Input: part model. Units: mm. Frame: model coordinates. Face numbers are marked on the shaded views. A direction names the side the tool comes from. Round coordinates to 2 decimals unless told otherwise and drop trailing zeros. Loops run counter-clockwise (first coordinate to the right, second up) from the corner with the lowest first, then second, coordinate; pieces in that order, holes last.
(1) Cut plane A-A, the plane y = 22. Output: boundary loops of the cut face in (x, z), and give its area (3 significant figures).
(2) Line query: line 1 (X direction, y = 32.75, z = 5); line 2 (Z direction, x = 0, y = 39); line 3 (Y direction, x = -48, z = 10). Output: solid intervals per line, ascending.
(3) Draft query along Z for the marked faces 1, 2, 3 and 4. Return one class per face: released by +Z, released by -Z, zero draft, split by the parting line, or undercut.
(4) First-contact query: pin 1 Ø12.5 at (x, y) = (-34.5, 28) entering from -Z; pin 2 Ø3 at (x, z) = (-34.25, -5) entering from -Y; pin 3 Ø6.5 at (x, y) = (13.5, 17.5) entering from -Z. Flat tips, straight axial feed; report the tip coordinate or a pass-through.
(5) Cut plane C-C, the plane y = 7. Output: boundary loops of the cut face in (x, z), and give its area (3 significant figures).
(6) Access query for the marked faces 5 and 6. Directions: +Z, -Z, +X, -X, +Y, -Y. A direction counts if a zero-diameter tool reaches every point of the face in a straight line with its end or side. Return the directions, or none.
(7) Cut plane B-B, the plane x = 0. Output: boundary loops of the cut face in (y, z) (3 decimals).
(8) Cut plane D-D, the plane y = 51. Output: boundary loops of the cut face in (x, z).
from build123d import *

# Parameters (mm, degrees)
SKETCH1_R                                           = 60.625
SKETCH1_R_2                                         = 45
BOSS_EXTRUDE1_DEPTH                                 = 4
SKETCH2_R                                           = 49
SKETCH2_R_2                                         = 45
BOSS_EXTRUDE2_DEPTH                                 = 52
SKETCH4_W                                           = 13.25
SKETCH4_H                                           = 8
SKETCH4_W_2                                         = 8
SKETCH4_H_2                                         = 38
BOSS_EXTRUDE4_DEPTH                                 = 13
BOSS_EXTRUDE5_DEPTH                                 = 4
SKETCH7_R                                           = 1.3
CUT_EXTRUDE4_DEPTH                                  = 7.2
SKETCH9_W                                           = 10
SKETCH9_H                                           = 24
CUT_EXTRUDE7_DEPTH                                  = 8
CUT_EXTRUDE8_REACH                                  = 111.625
SKETCH11_R                                          = 5
CUT_EXTRUDE9_DEPTH                                  = 5.0000001
CSK_FOR_M3_COUNTERSUNK_FLAT_HEAD_SCREW1_D           = 3.4
CSK_FOR_M3_COUNTERSUNK_FLAT_HEAD_SCREW1_DEPTH       = 4
CSK_FOR_M3_COUNTERSUNK_FLAT_HEAD_SCREW1_CSINK_D     = 6.3
CSK_FOR_M3_COUNTERSUNK_FLAT_HEAD_SCREW1_CSINK_ANGLE = 90


with BuildPart() as part:
    # Sketch1 → Boss-Extrude1 (new body)
    with BuildSketch(Plane(origin=(0, 0, 0), x_dir=(1, 0, 0), z_dir=(0, 1, 0))):
        Circle(SKETCH1_R)
        Circle(SKETCH1_R_2, mode=Mode.SUBTRACT)
    extrude(amount=BOSS_EXTRUDE1_DEPTH)

    # Sketch2 → Boss-Extrude2 (add)
    with BuildSketch(Plane(origin=(0, 4, 0), x_dir=(1, 0, 0), z_dir=(0, 1, 0))):
        Circle(SKETCH2_R)
        Circle(SKETCH2_R_2, mode=Mode.SUBTRACT)
    extrude(amount=BOSS_EXTRUDE2_DEPTH)

    # Sketch4 → Boss-Extrude4 (add, symmetric)
    with BuildSketch(Plane.XY):
        with Locations((-38.375, 34)):
            Rectangle(SKETCH4_W, SKETCH4_H)
        Polygon((-31.75, 30), (-45, 30), (-45, 16.75), align=None)
        with Locations((15.25, 19)):
            Rectangle(SKETCH4_W_2, SKETCH4_H_2)
    extrude(amount=BOSS_EXTRUDE4_DEPTH, both=True)

    # Sketch5 → Boss-Extrude5 (add)
    with BuildSketch(Plane.XZ):
        with BuildLine():
            Line((11.25, 13), (29.067400866, 34.352382842))
            ThreePointArc((29.067400866, 34.352382842), (45, 0), (29.067400866, -34.352382842))
            Line((29.067400866, -34.352382842), (11.25, -13))
            Line((11.25, -13), (11.25, 13))
        make_face()
    extrude(amount=-BOSS_EXTRUDE5_DEPTH)

    # Sketch7 → Cut-Extrude4 (cut)
    with BuildSketch(Plane(origin=(0, 38, 0), x_dir=(1, 0, 0), z_dir=(0, 1, 0))):
        with Locations((-34.25, 5)):
            Circle(SKETCH7_R)
        with Locations((-34.25, -5)):
            Circle(SKETCH7_R)
        with Locations((13.75, 5)):
            Circle(SKETCH7_R)
        with Locations((13.75, -5)):
            Circle(SKETCH7_R)
    extrude(amount=-CUT_EXTRUDE4_DEPTH, mode=Mode.SUBTRACT)

    # Sketch9 → Cut-Extrude7 (cut)
    with BuildSketch(Plane.ZY.offset(-11.25)):
        with Locations((0, 17)):
            Rectangle(SKETCH9_W, SKETCH9_H)
    extrude(amount=-CUT_EXTRUDE7_DEPTH, mode=Mode.SUBTRACT)

    # Sketch11 → Cut-Extrude8 (cut, up to next)
    with BuildSketch(Plane(origin=(49, 0, 0), x_dir=(0, 0, -1), z_dir=(1, 0, 0)), mode=Mode.PRIVATE) as cut_extrude8_sk1:
        with Locations((0, 14)):
            Circle(SKETCH11_R)
    cut_extrude8_tool1 = extrude(cut_extrude8_sk1.sketch, amount=-CUT_EXTRUDE8_REACH, mode=Mode.PRIVATE) & part.part
    add(cut_extrude8_tool1.solids().sort_by_distance((49, 14, 0))[0], mode=Mode.SUBTRACT)

    # Sketch12 → Cut-Extrude9 (cut, through all)
    with BuildSketch(Plane(origin=(0, 4, 0), x_dir=(1, 0, 0), z_dir=(0, 1, 0))):
        with BuildLine():
            Line((29.479537487, 22.359715328), (27.25, 19.687836398))
            Line((27.25, 19.687836398), (27.25, -19.687836398))
            Line((27.25, -19.687836398), (29.479537487, -22.359715328))
            ThreePointArc((29.479537487, -22.359715328), (37, 0), (29.479537487, 22.359715328))
        make_face()
        Polygon((27.25, -19.687836398), (27.25, 19.687836398), (24.25, 16.092634774), (24.25, -16.092634774), align=None)
    extrude(amount=-CUT_EXTRUDE9_DEPTH, mode=Mode.SUBTRACT)

    # CSK for M3 Countersunk Flat Head Screw1
    with Locations(Plane(origin=(0, 4, 0), x_dir=(1, 0, 0), z_dir=(0, 1, 0))):
        with Locations((-38.890872965, 38.890872965), (-38.890872965, -38.890872965), (38.890872965, -38.890872965), (38.890872965, 38.890872965)):
            CounterSinkHole(CSK_FOR_M3_COUNTERSUNK_FLAT_HEAD_SCREW1_D / 2, CSK_FOR_M3_COUNTERSUNK_FLAT_HEAD_SCREW1_CSINK_D / 2, depth=CSK_FOR_M3_COUNTERSUNK_FLAT_HEAD_SCREW1_DEPTH, counter_sink_angle=CSK_FOR_M3_COUNTERSUNK_FLAT_HEAD_SCREW1_CSINK_ANGLE)


solid = part.part
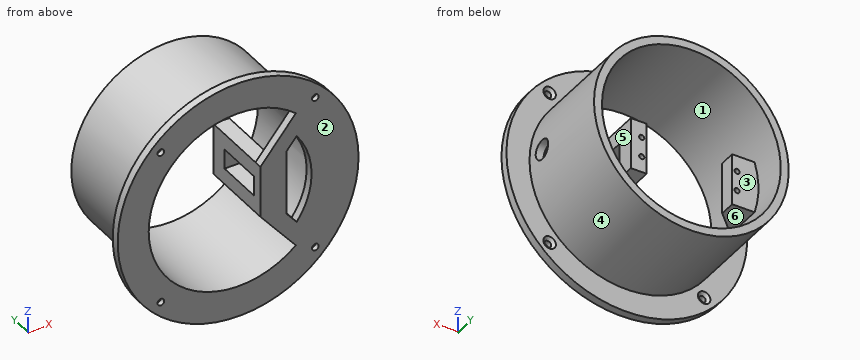
Reported:
1. outline: circle Ø98 at (0, 0); (11.25, -13) - (19.25, -13) - (19.25, -5) - (11.25, -5) - close; (11.25, 5) - (19.25, 5) - (19.25, 13) - (11.25, 13) - close; hole (-43.08, -13) arc R45 ccw (long way) to (-43.08, 13) - (-39.75, 13) - (-39.75, -13) - close
1. area: 1,430 mm2
2. line 1: x = -48.74 to -35.55, -32.95 to -31.75, 11.25 to 12.45, 15.05 to 19.25, 44.72 to 48.74
2. line 2: z = -49 to -45, 45 to 49
2. line 3: y = 0 to 4
3. face 1: undercut
3. face 2: zero draft
3. face 3: undercut
3. face 4: split by the parting line
4. pin 1: stops at z = -40.04
4. pin 2: stops at y = 26
4. pin 3: stops at z = -47.92
5. outline: circle Ø98 at (0, 0); (11.25, -13) - (19.25, -13) - (19.25, -5) - (11.25, -5) - close; (11.25, 5) - (19.25, 5) - (19.25, 13) - (11.25, 13) - close; hole circle Ø90 at (0, 0)
5. area: 1,310 mm2
6. face 5: +Y
6. face 6: +Y, -Y
7. outline: (0, -60.625) - (4, -60.625) - (4, -49) - (56, -49) - (56, -45) - (0, -45) - close; (0, 45) - (56, 45) - (56, 49) - (4, 49) - (4, 60.625) - (0, 60.625) - close
8. outline: circle Ø98 at (0, 0); hole circle Ø90 at (0, 0)
